```python
from build123d import *

# Parameters (mm, degrees)
AUFSATZ_LINEAR_AUSTRAGEN1_DEPTH = 550
SCHNITT_LINEAR_AUSTRAGEN1_DEPTH = 140


with BuildPart() as part:
    # Skizze1 → Aufsatz-Linear austragen1 (new, symmetric)
    with BuildSketch(Plane.XY):
        with BuildLine():
            Line((-34, 40), (34, 40))
            ThreePointArc((34, 40), (38.242640687, 38.242640687), (40, 34))
            Line((40, 34), (40, -34))
            ThreePointArc((40, -34), (38.242640687, -38.242640687), (34, -40))
            Line((34, -40), (-34, -40))
            ThreePointArc((-34, -40), (-38.242640687, -38.242640687), (-40, -34))
            Line((-40, -34), (-40, 34))
            ThreePointArc((-40, 34), (-38.242640687, 38.242640687), (-34, 40))
        make_face()
        with BuildLine():
            Line((-37, 34), (-37, -34))
            ThreePointArc((-37, -34), (-36.121320344, -36.121320344), (-34, -37))
            Line((-34, -37), (34, -37))
            ThreePointArc((34, -37), (36.121320344, -36.121320344), (37, -34))
            Line((37, -34), (37, 34))
            ThreePointArc((37, 34), (36.121320344, 36.121320344), (34, 37))
            Line((34, 37), (-34, 37))
            ThreePointArc((-34, 37), (-36.121320344, 36.121320344), (-37, 34))
        make_face(mode=Mode.SUBTRACT)
    extrude(amount=AUFSATZ_LINEAR_AUSTRAGEN1_DEPTH, both=True)

    # Skizze2 → Schnitt-Linear austragen1 (cut)
    with BuildSketch(Plane(origin=(0, 40, 0), x_dir=(1, 0, 0), z_dir=(0, 1, 0))):
        Polygon((-40, 550), (40, 550), (40, 470), align=None)
        Polygon((40, -470), (-40, -550), (40, -550), align=None)
    extrude(amount=-SCHNITT_LINEAR_AUSTRAGEN1_DEPTH, mode=Mode.SUBTRACT)


solid = part.part
```
Check sheet for the modelled part. Datum: model origin and axes. Units: mm. A direction names the side the tool comes from. Coordinates: 2 decimals unless noted, no trailing zeros. Order: outer loops, then holes, each group sorted by start corner. A loop starts at its lowest first (then second) coordinate and runs counter-clockwise, first axis right, second up. Notation, with made-up numbers: M 26,25 L 62,25 A8 cw 62,38 Z; hole C 76,50 d3. An arc over 180 degrees is marked long. One line per question, with ' | ' between items. Start each with the question number.
Item 1: Sectioned sample at A-A on x = 24. Record the cut outline in (y, z), and give its area (3 significant figures).
Item 2: Sectioned sample at B-B on y = -6.5. Record the cut outline in (x, z), and give its area (3 significant figures).
Item 3: Gauge pin test, flat end, axial feed: P1, Ø8, axis at x = -13.5, y = -30.5, coming from the +Z side. Record the tip position at first contact, or that the pin passes through.
Item 4: Material ranges on line 1 (Y direction, x = 29.5, z = -456); line 2 (X direction, y = 35, z = -0.5), recorded low to high.
Item 5: Access from +Z, -Z, +X, -X, +Y, -Y to the whole of each face (thin tool, end or side, straight path). Record for faces 4 (the flat face through (40, 0, 7)), 5 (the flat face through (0, -37, 8)).
Item 6: Mould release check, pull along X, two halves, no side actions. Record for faces 1 (the flat face through (0, 39, 510)), 2 (the flat face through (0, -40, 8)), 3 (the flat face through (0, 37, 8)): pulls with the +X half, pulls with the -X half, needs draft (parallel to the pull), parting line crosses it, or undercut.
Item 7: Sectioned sample at C-C on z = 451. Record the cut outline in (x, y).
Answer below:
1) outline: M -40,-486 L -37,-486 L -37,486 L -40,486 Z; M 37,-486 L 40,-486 L 40,486 L 37,486 Z | area: 5,830 mm^2
2) outline: M -40,-550 L -37,-547 L -37,547 L -40,550 Z; M 37,-473 L 40,-470 L 40,470 L 37,473 Z | area: 6,120 mm^2
3) P1: passes through
4) line 1: y = -40 to -37, 37 to 40 | line 2: x = -39.92 to -36.83, 36.83 to 39.92
5) face 4: +Z, -Z, +X, +Y, -Y | face 5: +Z, -Z
6) face 1: pulls with the +X half | face 2: needs draft | face 3: undercut
7) outline: M -40,-34 A6 ccw -34,-40 L 34,-40 A6 ccw 40,-34 L 40,34 A6 ccw 34,40 L -34,40 A6 ccw -40,34 Z; hole M -37,-34 A3 ccw -34,-37 L 34,-37 A3 ccw 37,-34 L 37,34 A3 ccw 34,37 L -34,37 A3 ccw -37,34 Z
